```python
from build123d import *

# Parameters (mm, degrees)
SKETCH_1_R          = 15
EXTRUDE_1_DEPTH     = 3
CUT_EXTRUDE_1_REACH = 23.424
SKETCH_2_R          = 5
CUT_EXTRUDE_2_REACH = 23.424
SKETCH_3_R          = 1.8


with BuildPart() as part:
    # 草图1 → 凸台-拉伸1 (new body)
    with BuildSketch(Plane.XY):
        Circle(SKETCH_1_R)
    extrude(amount=EXTRUDE_1_DEPTH)

    # 草图2 → 切除-拉伸1 (cut, up to next)
    with BuildSketch(Plane.XY.offset(3), mode=Mode.PRIVATE) as cut_extrude_1_sk1:
        Circle(SKETCH_2_R)
    cut_extrude_1_tool1 = extrude(cut_extrude_1_sk1.sketch, amount=-CUT_EXTRUDE_1_REACH, mode=Mode.PRIVATE) & part.part
    add(cut_extrude_1_tool1.solids().sort_by_distance((0, 0, 3))[0], mode=Mode.SUBTRACT)

    # 草图3 → 切除-拉伸2 (cut, up to next)
    with BuildSketch(Plane.XY.offset(3), mode=Mode.PRIVATE) as cut_extrude_2_sk1:
        with Locations((-10.356157589, -7)):
            Circle(SKETCH_3_R)
    cut_extrude_2_tool1 = extrude(cut_extrude_2_sk1.sketch, amount=-CUT_EXTRUDE_2_REACH, mode=Mode.PRIVATE) & part.part
    # 草图3 → 切除-拉伸2 (cut, up to next)
    with BuildSketch(Plane.XY.offset(3), mode=Mode.PRIVATE) as cut_extrude_2_sk2:
        with Locations((10.356157589, -7)):
            Circle(SKETCH_3_R)
    cut_extrude_2_tool2 = extrude(cut_extrude_2_sk2.sketch, amount=-CUT_EXTRUDE_2_REACH, mode=Mode.PRIVATE) & part.part
    # 草图3 → 切除-拉伸2 (cut, up to next)
    with BuildSketch(Plane.XY.offset(3), mode=Mode.PRIVATE) as cut_extrude_2_sk3:
        with Locations((10.356157589, 7)):
            Circle(SKETCH_3_R)
    cut_extrude_2_tool3 = extrude(cut_extrude_2_sk3.sketch, amount=-CUT_EXTRUDE_2_REACH, mode=Mode.PRIVATE) & part.part
    # 草图3 → 切除-拉伸2 (cut, up to next)
    with BuildSketch(Plane.XY.offset(3), mode=Mode.PRIVATE) as cut_extrude_2_sk4:
        with Locations((-10.356157589, 7)):
            Circle(SKETCH_3_R)
    cut_extrude_2_tool4 = extrude(cut_extrude_2_sk4.sketch, amount=-CUT_EXTRUDE_2_REACH, mode=Mode.PRIVATE) & part.part
    add(cut_extrude_2_tool1.solids().sort_by_distance((-10.356158, -7, 3))[0], mode=Mode.SUBTRACT)
    add(cut_extrude_2_tool2.solids().sort_by_distance((10.356158, -7, 3))[0], mode=Mode.SUBTRACT)
    add(cut_extrude_2_tool3.solids().sort_by_distance((10.356158, 7, 3))[0], mode=Mode.SUBTRACT)
    add(cut_extrude_2_tool4.solids().sort_by_distance((-10.356158, 7, 3))[0], mode=Mode.SUBTRACT)


solid = part.part
```
Design review of the part built by this model. Coordinates are the model's own, in mm. Coordinates: 2 decimals unless noted, no trailing zeros. Order: outer loops, then holes, each group sorted by start corner. A loop starts at its lowest first (then second) coordinate and runs counter-clockwise, first axis right, second up. Notation, with made-up numbers: (-21.5, 81) - (19.5, 81) arc R26 ccw to (19.5, 107) - close; hole circle Ø5 at (26, 70.5). An arc over 180 degrees is marked (long way). Answer in a Markdown table with one row per item.
(1) Consider section D-D on x = -9.5. State the section outline as (y, z) points, plus the area to 3 significant figures.
Checked values:
| item | result |
|---|---|
| outline | (-11.61, 0) - (-8.58, 0) - (-8.58, 3) - (-11.61, 3) - close; (-5.42, 0) - (5.42, 0) - (5.42, 3) - (-5.42, 3) - close; (8.58, 0) - (11.61, 0) - (11.61, 3) - (8.58, 3) - close |
| area | 50.6 mm^2 |
(2) Consider section A-A on x = 0. State the section outline as (y, z) points, plus the area to 3 significant figures.
Checked values:
| item | result |
|---|---|
| outline | (-15, 0) - (-5, 0) - (-5, 3) - (-15, 3) - close; (5, 0) - (15, 0) - (15, 3) - (5, 3) - close |
| area | 60.0 mm^2 |
(3) Clearance check with flat-ended pins moving along their axes: pin 1 (3 mm diameter, centred on x = -10.36, y = 7, fed in from -Z); pin 2 (1.5 mm diameter, centred on x = -6.5, z = 1.5, fed in from +Y); pin 3 (1.5 mm diameter, centred on x = 5.5, z = 2.5, fed in from +Y). State where each tip first meets the part, or that it passes through.
Checked values:
| item | result |
|---|---|
| pin 1 | through |
| pin 2 | y = 13.85 |
| pin 3 | y = 14.23 |
(4) Consider section B-B on y = 2.25. State the section outline as (x, z) points, plus the area to 3 significant figures.
Checked values:
| item | result |
|---|---|
| outline | (-14.83, 0) - (-4.47, 0) - (-4.47, 3) - (-14.83, 3) - close; (4.47, 0) - (14.83, 0) - (14.83, 3) - (4.47, 3) - close |
| area | 62.2 mm^2 |
(5) Wall thickness on line 1 along Y through (x, z) = (0, 1.1); line 2 along Y through (x, z) = (-12, 2.4); line 3 along X through (y, z) = (-6.5, 2): over which ranges is each line inside the solid? List them lowest first. Write a range as from..to.
Checked values:
| item | result |
|---|---|
| line 1 | -15..-5, 5..15 |
| line 2 | -9..-7.73, -6.27..6.27, 7.73..9 |
| line 3 | -13.52..-12.09, -8.63..8.63, 12.09..13.52 |
(6) The part is to be moulded in two halves that separate along Y. For faces 1 (the flat face through (-4, 4, 3)), 2 (the cylindrical face through (-14.985, 0.66, 1.479)), 3 (the cylindrical face through (12.02, -7.69, 1.52)), say which applies: released by +Y, released by -Y, zero draft, split by the parting line, or undercut.
Checked values:
| item | result |
|---|---|
| face 1 | zero draft |
| face 2 | split by the parting line |
| face 3 | undercut |
(7) Consider section C-C on z = 1. State the section outline as (x, y) points.
Checked values:
| item | result |
|---|---|
| outline | circle Ø30 at (0, 0); hole circle Ø3.6 at (-10.36, -7); hole circle Ø3.6 at (-10.36, 7); hole circle Ø10 at (0, 0); hole circle Ø3.6 at (10.36, -7); hole circle Ø3.6 at (10.36, 7) |
